Read the model definition and answer for the solid it produces. Units are mm, in the model's axes. Give positions to 0.01 mm unless a question says otherwise; leave off trailing zeros. Order: outer loops, then holes, each group sorted by start corner. A loop starts at its lowest first (then second) coordinate and runs counter-clockwise, first axis right, second up.
Item 1: A cutting plane is placed at B-B (y = 0). Write down the section's boundary in (x, z).
Item 2: Given pin 1 Ø2.5 at (y, z) = (-18.5, 3.5) entering from +X; pin 2 Ø19.5 at (x, y) = (-59.3, 0) entering from -Z; pin 3 Ø12 at (x, y) = (60.7, 0) entering from -Z; pin 4 Ø1.5 at (y, z) = (-17.5, 3.5) entering from -X, each flat-ended and moving along its own axis, determine where each tip first touches the part or whether it passes through.
Item 3: A cutting plane is placed at C-C (z = 2.5). State how many separate pieces and enclosed holes the cut face has, plus the area to 3 significant figures.
Item 4: A cutting plane is placed at D-D (x = -59.3). Write down the section's boundary in (y, z).
Item 5: Find the intervals of material crossed by line 1 along Y through (x, z) = (60.7, 2.85); line 2 along Y through (x, z) = (-59.3, 2.7); line 3 along X through (y, z) = (-2.5, 3.8), in increasing order.
Item 6: A cutting plane is placed at A-A (x = 60.7). Write down the section's boundary in (y, z).
Autodesk Inventor part; units mm, degrees
ref_plane "YZ Plane" through (0, 0, 0) normal (1, 0, 0) x (0, 1, 0)
ref_plane "XZ Plane" through (0, 0, 0) normal (0, 1, 0) x (-1, 0, 0)
ref_plane "XY Plane" through (0, 0, 0) normal (0, 0, 1) x (1, 0, 0)
sketch "Sketch1" plane through (0, 0, 0) normal (0, 0, 1) x (1, 0, 0)
  line L0 (-195, 15) -> (195, 15)
  line L1 (195, 15) -> (195, -15)
  line L2 (195, -15) -> (-195, -15)
  line L3 (-195, -15) -> (-195, 15)
  line L4 (-195, 15) -> (195, -15) construction
  line L5 (195, 15) -> (-195, -15) construction
  point P0 (0, 0)
  dimension "d0" = 390
  dimension "d1" = 30
extrude "Base" add sketch "Sketch1" along normal blind 5
sketch "Sketch3" plane through (0, 0, 5) normal (0, 0, 1) x (1, 0, 0)
  circle A0 centre (60.7, 0) radius 7.5
  circle A1 centre (-59.3, 0) radius 7.5
  line L0 (195, -15) -> (195, 15)
  dimension "d16" = 15
  dimension "d17" = 15
  dimension "d20" = 134.3
  dimension "d22" = 120
extrude "Extrusion3" cut sketch "Sketch3" against normal blind 10
sketch "Sketch4" plane through (0, 0, 5) normal (0, 0, 1) x (1, 0, 0)
  line L0 (-195, -15) -> (195, -15)
  line L1 (165, -15) -> (145, -15)
  line L2 (145, -15) -> (145, -20)
  line L3 (145, -20) -> (165, -20)
  line L4 (165, -20) -> (165, -15)
  line L5 (115, -15) -> (95, -15)
  line L6 (95, -15) -> (95, -20)
  line L7 (95, -20) -> (115, -20)
  line L8 (115, -20) -> (115, -15)
  line L9 (65, -15) -> (45, -15)
  line L10 (45, -15) -> (45, -20)
  line L11 (45, -20) -> (65, -20)
  line L12 (65, -20) -> (65, -15)
  line L13 (15, -15) -> (-5, -15)
  line L14 (-5, -15) -> (-5, -20)
  line L15 (-5, -20) -> (15, -20)
  line L16 (15, -20) -> (15, -15)
  line L17 (-35, -15) -> (-55, -15)
  line L18 (-55, -15) -> (-55, -20)
  line L19 (-55, -20) -> (-35, -20)
  line L20 (-35, -20) -> (-35, -15)
  line L21 (-85, -15) -> (-105, -15)
  line L22 (-105, -15) -> (-105, -20)
  line L23 (-105, -20) -> (-85, -20)
  line L24 (-85, -20) -> (-85, -15)
  line L25 (-135, -15) -> (-155, -15)
  line L26 (-155, -15) -> (-155, -20)
  line L27 (-155, -20) -> (-135, -20)
  line L28 (-135, -20) -> (-135, -15)
  point P0 (0, 0)
  point P1 (-35, -15)
  point P2 (-55, -15)
  point P3 (-135, -15)
  point P4 (-155, -15)
  point P5 (115, -15)
  point P6 (95, -15)
  point P7 (-85, -15)
  point P8 (-105, -15)
  point P9 (65, -15)
  point P10 (45, -15)
  point P11 (15, -15)
  point P12 (-5, -15)
  point P13 (145, -15)
  dimension "d23" = 20
  dimension "d24" = 5
  dimension "d25" = 30
  dimension "d28" = 50
extrude "Extrusion4" add sketch "Sketch4" against normal blind 5
properties part number "Divisória-30cm c rolamento"
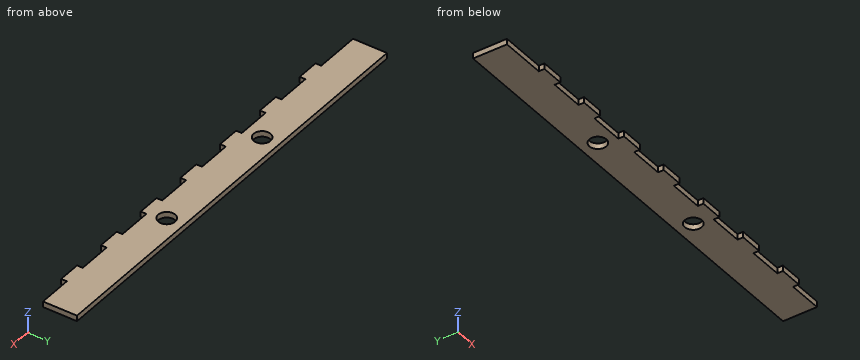
Response values:
1. outline: (-195, 0) - (-66.8, 0) - (-66.8, 5) - (-195, 5) - close; (-51.8, 0) - (53.2, 0) - (53.2, 5) - (-51.8, 5) - close; (68.2, 0) - (195, 0) - (195, 5) - (68.2, 5) - close
2. pin 1: stops at x = 165
2. pin 2: stops at z = 0
2. pin 3: passes through
2. pin 4: stops at x = -155
3. separate pieces: 1
3. enclosed holes: 2
3. area: 12,000 mm2
4. outline: (-15, 0) - (-7.5, 0) - (-7.5, 5) - (-15, 5) - close; (7.5, 0) - (15, 0) - (15, 5) - (7.5, 5) - close
5. line 1: y = -20 to -7.5, 7.5 to 15
5. line 2: y = -15 to -7.5, 7.5 to 15
5. line 3: x = -195 to -66.37, -52.23 to 53.63, 67.77 to 195
6. outline: (-20, 0) - (-7.5, 0) - (-7.5, 5) - (-20, 5) - close; (7.5, 0) - (15, 0) - (15, 5) - (7.5, 5) - close
